Verification items for this drawing (mm, ordinates from the low corner). Coordinates: 2 decimals unless noted, no trailing zeros. Write each loop counter-clockwise with the first axis right and the second up, starting at its lowest first coordinate (ties: lowest second). Pieces come first, ordered by that corner, then holes. Notation, with made-up numbers: (-14.75, 74.5) -> (0.25, 74.5) arc R27 cw to (0.25, 102.5) -> close; hole circle Ø2 at (8.25, 13). An arc over 180 degrees is marked (long way). Put each result on its own line as item: value. Start each with the question number.
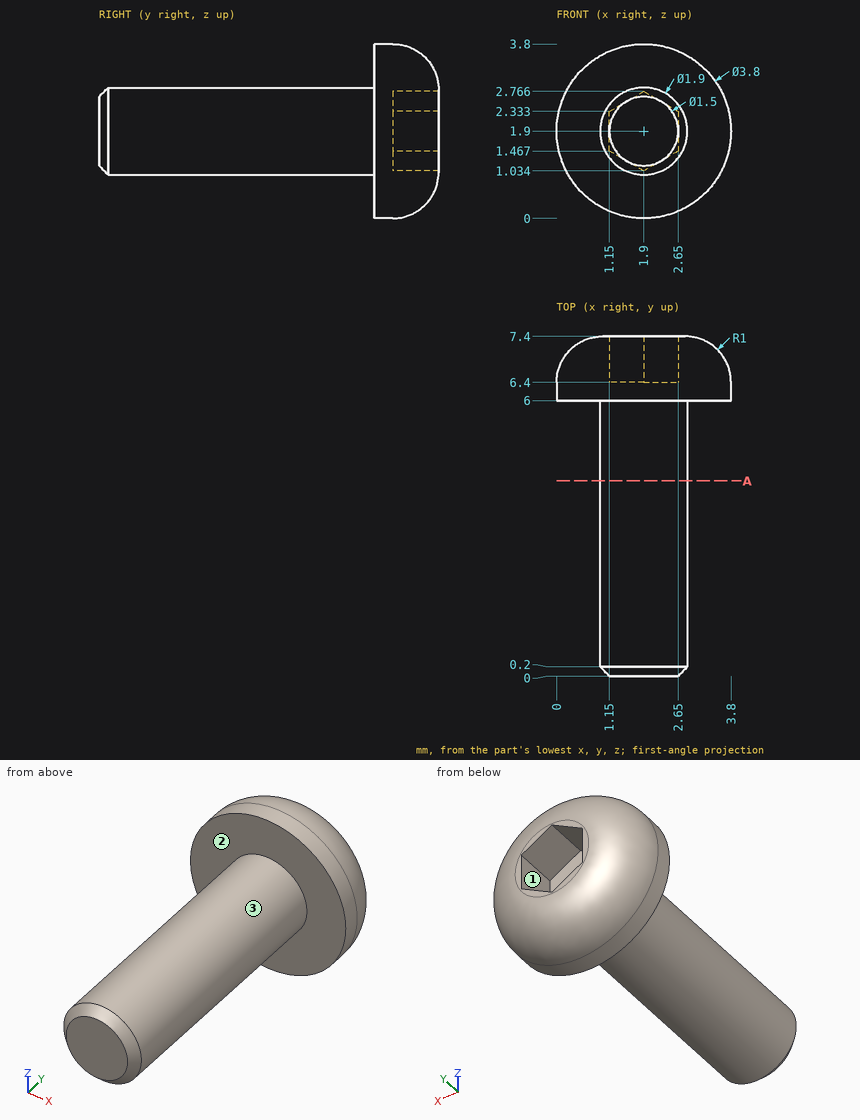
Item 1: Section check A-A, the plane y = 4.25. Enter the section's corners in (x, z).
Item 2: Scan lines: line 1 along Z through (x, y) = (1.7, 6.5); line 2 along X through (y, z) = (6.75, 1.85); line 3 along X through (y, z) = (1.25, 1.6). Record each from-to range of solid material in increasing order. Write a range as [from, to].
Item 3: Go/stop test with flat-tipped pins: P1, Ø2, axis at x = 3, y = 1, coming from the -Z side; P2, Ø1, axis at y = 3.5, z = 2.5, coming from the +X side. Record where each tip stops, or that it passes through.
Item 4: Mould release check, pull along Z, two halves, no side actions. Record for the marked faces 1, 2 and 3: released by +Z, released by -Z, zero draft, split by the parting line, or undercut.
From the geometry:
1. outline: circle Ø1.9 at (1.9, 1.9)
2. line 1: [0.02, 1.15], [2.65, 3.78]
2. line 2: [0.06, 1.15], [2.65, 3.74]
2. line 3: [1, 2.8]
3. P1: z = 0.96
3. P2: x = 2.84
4. face 1: undercut
4. face 2: zero draft
4. face 3: split by the parting line
